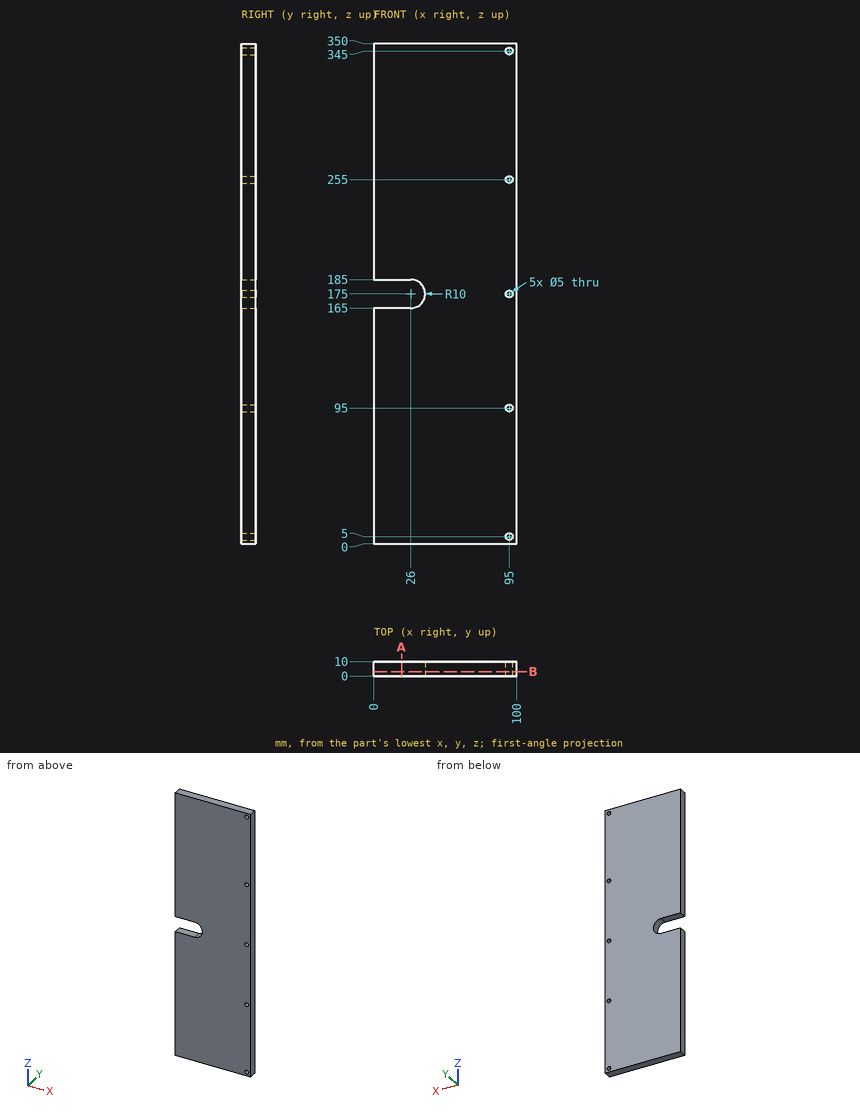
Answer from the drawing. Dimensions are ordinates in mm from the lowest x, y and z of the part. Coordinates: 2 decimals unless noted, no trailing zeros. Order: outer loops, then holes, each group sorted by start corner. A loop starts at its lowest first (then second) coordinate and runs counter-clockwise, first axis right, second up. Notation, with made-up numbers: (7.5, 47) - (55.5, 47) arc R38 ccw to (55.5, 86) - close; hole circle Ø2 at (-22, 34). An arc over 180 degrees is marked (long way). Answer as a JSON object with one key per item and string values. Group by question number.
Item 1: Section A-A (x = 19.5) is taken. Give the vertices of the cut face in (y, z).
Item 2: Consider probe 1 along Z at (x, y) = (95, 7); probe 2 along X at (y, z) = (2, 345); probe 3 along Z at (x, y) = (24.5, 9). Determine where each line is inside the solid, lowest interval first. Write a range as from..to.
Item 3: Flat-ended cylindrical pins translate along their axes: P1, Ø3, axis at x = 95, z = 255, coming from the -Y side; P2, Ø1, axis at y = 9, z = 169.5, coming from the -X side. Find the tip coordinate at first contact, or state that the pin passes through.
Item 4: Section B-B (y = 3) is taken. Give the vertices of the cut face in (x, z), plus the area to 3 significant figures.
Results are:
{
 "1": {"outline": "(0, 0) - (10, 0) - (10, 165) - (0, 165) - close; (0, 185) - (10, 185) - (10, 350) - (0, 350) - close"},
 "2": {"probe 1": "z = 0..2.5, 7.5..92.5, 97.5..172.5, 177.5..252.5, 257.5..342.5, 347.5..350", "probe 2": "x = 0..92.5, 97.5..100", "probe 3": "z = 0..165, 185..350"},
 "3": {"P1": "passes through", "P2": "stops at x = 34"},
 "4": {"outline": "(0, 0) - (100, 0) - (100, 350) - (0, 350) - (0, 185) - (26, 185) arc R10 cw to (26, 165) - (0, 165) - close; hole circle Ø5 at (95, 5); hole circle Ø5 at (95, 95); hole circle Ø5 at (95, 175); hole circle Ø5 at (95, 255); hole circle Ø5 at (95, 345)", "area": "34,200 mm^2"}
}
